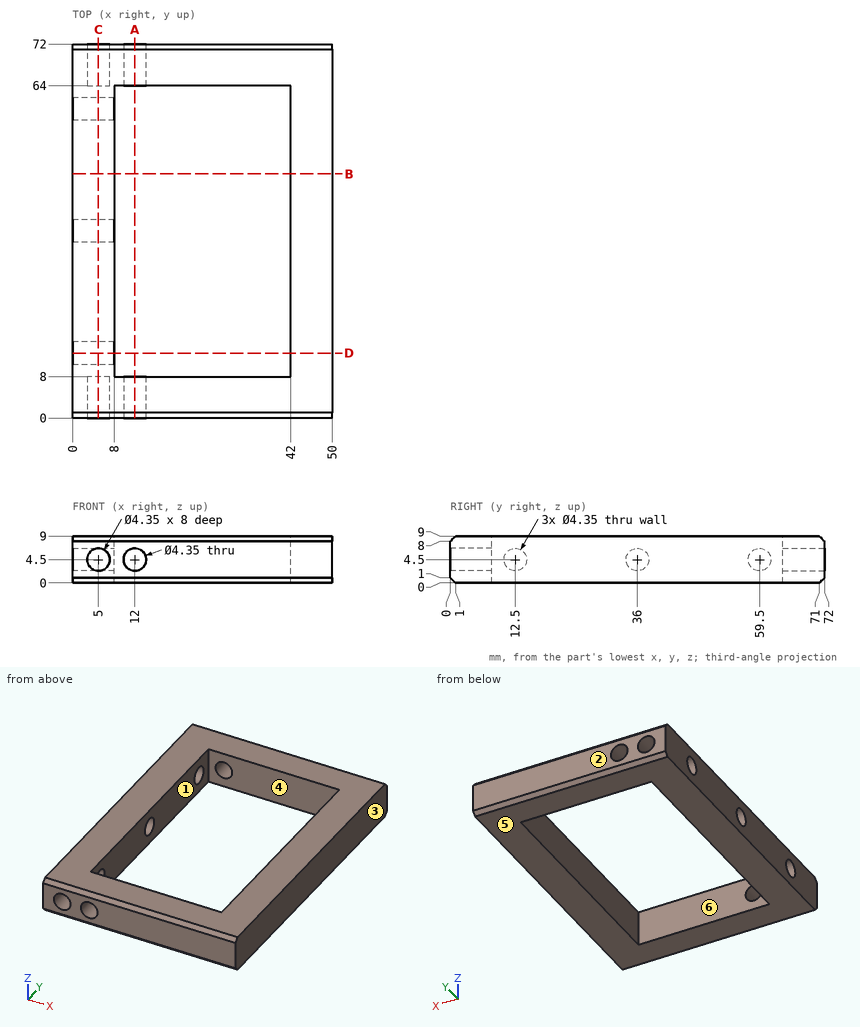
Source: three-view drawing plus pictorial views. Frame: mm from the lowest corner of the part. A direction names the side the tool comes from. Give positions to 0.01 mm unless a question says otherwise; leave off trailing zeros. Order: outer loops, then holes, each group sorted by start corner. A loop starts at its lowest first (then second) coordinate and runs counter-clockwise, first axis right, second up. Notation, with made-up numbers: M 41,71 L 73,71 A3 ccw 73,75 Z; hole C -33.5,87 d4. An arc over 180 degrees is marked long. Return JSON: item names as keys, results as strings.
1) Mould query, pull axis Y, two halves, no side actions, for the marked faces 1, 2, 3 and 4. Classes: released by +Y, released by -Y, zero draft, split by the parting line, or undercut.
Taken from the geometry:
{"face 1": "undercut", "face 2": "released by +Y", "face 3": "zero draft", "face 4": "undercut"}
2) Section query B-B on y = 47. Output: boundary loops of the cut face in (x, z).
Taken from the geometry:
{"outline": "M 0,0 L 8,0 L 8,9 L 0,9 Z; M 42,0 L 50,0 L 50,9 L 42,9 Z"}
3) Section query D-D on y = 12.5. Output: boundary loops of the cut face in (x, z) (3 decimals), and give its area (3 significant figures).
Taken from the geometry:
{"outline": "M 0,0 L 8,0 L 8,2.325 L 0,2.325 Z; M 0,6.675 L 8,6.675 L 8,9 L 0,9 Z; M 42,0 L 50,0 L 50,9 L 42,9 Z", "area": "109 mm2"}
4) Section query C-C on x = 5. Output: boundary loops of the cut face in (y, z) (3 decimals).
Taken from the geometry:
{"outline": "M 0,1 L 1,0 L 71,0 L 72,1 L 72,2.325 L 64,2.325 L 64,6.675 L 72,6.675 L 72,8 L 71,9 L 1,9 L 0,8 L 0,6.675 L 8,6.675 L 8,2.325 L 0,2.325 Z; hole C 12.5,4.5 d4.35; hole C 36,4.5 d4.35; hole C 59.5,4.5 d4.35"}
5) Line query: L1, parallel to Z at x = 5, y = 68.5 (3 decimals); L2, parallel to Y at x = 18, z = 2; L3, parallel to X at y = 49, z = 8.5. Output: solid intervals per line, ascending. Write a range as [from, to].
Taken from the geometry:
{"L1": "z = [0, 2.325], [6.675, 9]", "L2": "y = [0, 8], [64, 72]", "L3": "x = [0, 8], [42, 50]"}
6) Access query for the marked faces 5 and 6. Directions: +Z, -Z, +X, -X, +Y, -Y. A direction counts if a zero-diameter tool reaches every point of the face in a straight line with its end or side. Return the directions, or none.
Taken from the geometry:
{"face 5": "-Z, +X, -X, +Y, -Y", "face 6": "+Z, -Z"}
7) Section query A-A on x = 12. Output: boundary loops of the cut face in (y, z) (3 decimals), and give its area (3 significant figures).
Taken from the geometry:
{"outline": "M 0,1 L 1,0 L 8,0 L 8,2.325 L 0,2.325 Z; M 0,6.675 L 8,6.675 L 8,9 L 1,9 L 0,8 Z; M 64,0 L 71,0 L 72,1 L 72,2.325 L 64,2.325 Z; M 64,6.675 L 72,6.675 L 72,8 L 71,9 L 64,9 Z", "area": "72.4 mm2"}
8) Contact query for flat-ended pins moving along their axis: pin 1 (2.5 mm diameter, centred on x = 5, z = 4.5, fed in from -Y); pin 2 (2.5 mm diameter, centred on y = 12.5, z = 4.5, fed in from -X); pin 3 (1.3 mm diameter, centred on x = 5.5, z = 3.5, fed in from +Y). Output: stop coordinate, or through.
Taken from the geometry:
{"pin 1": "stops at y = 8", "pin 2": "stops at x = 42", "pin 3": "stops at y = 64"}
